```python
from build123d import *

# Parameters (mm, degrees)
SKETCH1_W                     = 130
SKETCH1_H                     = 32
BOSS_EXTRUDE1_DEPTH           = 32.131
SKETCH2_R                     = 6.5
CUT_EXTRUDE1_DEPTH            = 138.68224708
SKETCH3_R                     = 6.5
CUT_EXTRUDE2_DEPTH            = 12
TAP_DRILL_FOR_M12X1_75_TAP1_D = 10.2
CUT_EXTRUDE3_START            = -32.131
SKETCH10_W                    = 72.5
SKETCH10_H                    = 32
CUT_EXTRUDE3_DEPTH            = 1.85
CHAMFER1_SIZE                 = 3
CHAMFER1_SIZE2                = 1.732050808
BOSS_EXTRUDE2_DEPTH           = 10
SKETCH13_W                    = 1
SKETCH13_H                    = 1


with BuildPart() as part:
    # Sketch1 → Boss-Extrude1 (new body)
    with BuildSketch(Plane(origin=(0, 0, 0), x_dir=(1, 0, 0), z_dir=(0, 1, 0))):
        with Locations((65, 16)):
            Rectangle(SKETCH1_W, SKETCH1_H)
    extrude(amount=BOSS_EXTRUDE1_DEPTH)

    # Sketch2 → Cut-Extrude1 (cut, through all)
    with BuildSketch(Plane(origin=(0, 32.131, 0), x_dir=(1, 0, 0), z_dir=(0, 1, 0))):
        with Locations(Location((14.85, 16, 0), (0, 0, 270))):
            Circle(SKETCH2_R)
        with Locations(Location((39.85, 16, 0), (0, 0, 270))):
            Circle(SKETCH2_R)
    extrude(amount=-CUT_EXTRUDE1_DEPTH, mode=Mode.SUBTRACT)

    # Sketch3 → Cut-Extrude2 (cut)
    with BuildSketch(Plane(origin=(0, 32.131, 0), x_dir=(1, 0, 0), z_dir=(0, 1, 0))):
        with Locations(Location((115.1, 16, 0), (0, 0, 270))):
            Circle(SKETCH3_R)
    extrude(amount=-CUT_EXTRUDE2_DEPTH, mode=Mode.SUBTRACT)

    # Tap Drill for M12x1.75 Tap1 (through all)
    with Locations(Plane(origin=(0, 20.131, 0), x_dir=(1, 0, 0), z_dir=(0, 1, 0))):
        with Locations((115.1, 16)):
            Hole(TAP_DRILL_FOR_M12X1_75_TAP1_D / 2)

    # Sketch10 → Cut-Extrude3 (cut)
    with BuildSketch(Plane(origin=(0, 32.131, 0), x_dir=(1, 0, 0), z_dir=(0, 1, 0)).offset(CUT_EXTRUDE3_START)):
        with Locations((93.75, 16)):
            Rectangle(SKETCH10_W, SKETCH10_H)
    extrude(amount=CUT_EXTRUDE3_DEPTH, mode=Mode.SUBTRACT)

    # Chamfer1
    chamfer1_edges = [part.edges().sort_by_distance(p)[0] for p in [
        (57.5, 0, -16),
    ]]
    chamfer1_side = [part.faces().sort_by_distance(p)[0] for p in [
        (28.986038139, 0, -16),
    ]]
    chamfer(chamfer1_edges, length=CHAMFER1_SIZE, length2=CHAMFER1_SIZE2, reference=chamfer1_side[0])

    # Sketch12 → Boss-Extrude2 (add)
    with BuildSketch(Plane.ZY):
        Polygon((-20, 12.601398385), (-20, 19.529601615), (-26, 22.99370323), (-32, 19.529601615), (-32, 12.601398385), (-26, 9.13729677), align=None)
    extrude(amount=BOSS_EXTRUDE2_DEPTH)

    # Sketch13 → Cut-Revolve1 (revolve, cut)
    with BuildSketch(Plane.XY.offset(-26)):
        with Locations((-0.5, 22.49370323)):
            Rectangle(SKETCH13_W, SKETCH13_H)
        with Locations((-5.5, 22.49370323)):
            Rectangle(SKETCH13_W, SKETCH13_H)
    revolve(axis=Axis((0, 16.0655, -26), (-1, 0, 0)), mode=Mode.SUBTRACT)

    # Sketch14 → Revolve2 (revolve)
    with BuildSketch(Plane.XY.offset(-26), mode=Mode.PRIVATE) as revolve2_sk:
        Polygon((-10, 21.8155), (-16, 19.8155), (-50, 19.8155), (-50, 16.0655), (-10, 16.0655), align=None)
    revolve(revolve2_sk.sketch.rotate(Axis((-50, 16.0655, -26), (1, 0, 0)), 90), axis=Axis((-50, 16.0655, -26), (1, 0, 0)))


solid = part.part
```
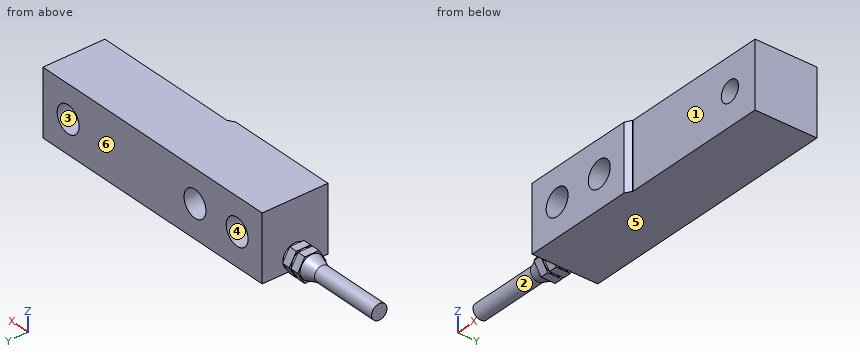
The model under review builds one solid part; all positions refer to its coordinate system, in mm. Face numbers are marked on the shaded views. A direction names the side the tool comes from. Coordinates: 2 decimals unless noted, no trailing zeros. Write each loop counter-clockwise with the first axis right and the second up, starting at its lowest first coordinate (ties: lowest second). Pieces come first, ordered by that corner, then holes.
1) We need section C-C on y = 7. State the section outline as (x, z) points, then the cut area to 3 significant figures.
2) Machinability: for the marked faces 1, 2 and 3, which of the approach directions +Z, -Z, +X, -X, +Y, -Y give a long, thin tool a straight path to every point of the face, cutting with its end or side? Answer none if there is none.
3) To check wall thickness, follow probe 1 along X at (y, z) = (20.5, -16); probe 2 along X at (y, z) = (28.5, -12); probe 3 along X at (y, z) = (6, -10). State the ranges of each line that lie inside material, in increasing order.
4) Clearance check with flat-ended pins moving along their axes: pin 1 Ø17 at (x, z) = (115.1, -16) entering from -Y; pin 2 Ø1.2 at (x, y) = (-2, 15.5) entering from +Z; pin 3 Ø11.5 at (x, z) = (39.85, -16) entering from +Y; pin 4 Ø6 at (y, z) = (6.5, -28) entering from -X. State where each tip first meets the part, or that it passes through.
5) We need section D-D on z = -3. State the section outline as (x, y) points.
6) We need section A-A on z = -16. State the section outline as (x, y) points.
7) The part is to be moulded in two halves that separate along Z. For the marked faces 4, 5 and 6, say which applies: pulls with the +Z half, pulls with the -Z half, needs draft (parallel to the pull), parting line crosses it, or undercut.
8) We need section B-B on x = 115.1. State the section outline as (y, z) points, then the cut area to 3 significant figures.
Answer list:
1. outline: (0, -32) - (130, -32) - (130, 0) - (0, 0) - close; hole circle Ø13 at (14.85, -16); hole circle Ø13 at (39.85, -16); hole circle Ø10.2 at (115.1, -16)
1. area: 3,810 mm2
2. face 1: +Z, -Z, +X, -Y
2. face 2: -X
2. face 3: +Y
3. probe 1: x = 0 to 8.35, 21.35 to 33.35, 46.35 to 108.6, 121.6 to 130
3. probe 2: x = 0 to 9.73, 19.97 to 34.73, 44.97 to 109.98, 120.22 to 130
3. probe 3: x = 0 to 12.35, 17.35 to 37.35, 42.35 to 130
4. pin 1: stops at y = 1.85
4. pin 2: stops at z = -20
4. pin 3: passes through
4. pin 4: stops at x = 0
5. outline: (0, 0) - (54.5, 0) - (57.5, 1.73) - (57.5, 1.85) - (130, 1.85) - (130, 32.13) - (0, 32.13) - close
6. outline: (0, 0) - (8.35, 0) - (8.35, 32.13) - (0, 32.13) - close; (21.35, 0) - (33.35, 0) - (33.35, 32.13) - (21.35, 32.13) - close; (46.35, 0) - (54.5, 0) - (57.5, 1.73) - (57.5, 1.85) - (110, 1.85) - (110, 20.13) - (108.6, 20.13) - (108.6, 32.13) - (46.35, 32.13) - close; (120.2, 1.85) - (130, 1.85) - (130, 32.13) - (121.6, 32.13) - (121.6, 20.13) - (120.2, 20.13) - close
7. face 4: undercut
7. face 5: pulls with the -Z half
7. face 6: needs draft
8. outline: (1.85, -32) - (32.13, -32) - (32.13, -22.5) - (20.13, -22.5) - (20.13, -21.1) - (1.85, -21.1) - close; (1.85, -10.9) - (20.13, -10.9) - (20.13, -9.5) - (32.13, -9.5) - (32.13, 0) - (1.85, 0) - close
8. area: 627 mm2
